The listing builds one solid part. Answer for the finished solid, in the listing's coordinates (mm). Face numbers are marked on the shaded views. A direction names the side the tool comes from. Round coordinates to 2 decimals unless told otherwise and drop trailing zeros. Write each loop counter-clockwise with the first axis right and the second up, starting at its lowest first coordinate (ties: lowest second). Pieces come first, ordered by that corner, then holes.
Item 1: For a pull along Z with two mould halves and no side action, classify the marked faces 3, 4 and 5 as +Z half, -Z half, draft (parallel to the pull), parting line (faces both ways), or undercut.
Item 2: Find section D-D on z = -3.5. Give the vertices of the cut face in (x, y), then the cut area to 3 significant figures.
Item 3: Find section C-C on x = 13. Give the vertices of the cut face in (y, z), then the cut area to 3 significant figures.
Item 4: Find section A-A on z = 0. Give the vertices of the cut face in (x, y) (3 decimals).
Item 5: Each of these flat-tipped pins is pushed along its axis until it touches: pin 1 (3 mm diameter, centred on y = 2.5, z = 3.5, fed in from -X); pin 2 (2 mm diameter, centred on x = 6.5, z = -2, fed in from +Y). Where does it stop, or does it pass through?
Item 6: A tool of negligible diameter and unlimited length cuts with its end or side. For the marked faces 1 and 2, from which of +Z, -Z, +X, -X, +Y, -Y can it reach the whole face along a straight path? Write none if from no direction.
Item 7: Find the intervals of material crossed by probe 1 along X at (y, z) = (3.3, 0) (3 decimals); probe 2 along Y at (x, z) = (9, -3); probe 3 along X at (y, z) = (4.25, -1.75), in increasing order.
Item 8: Find section B-B on y = 3.55. Give the vertices of the cut face in (x, z) (3 decimals).
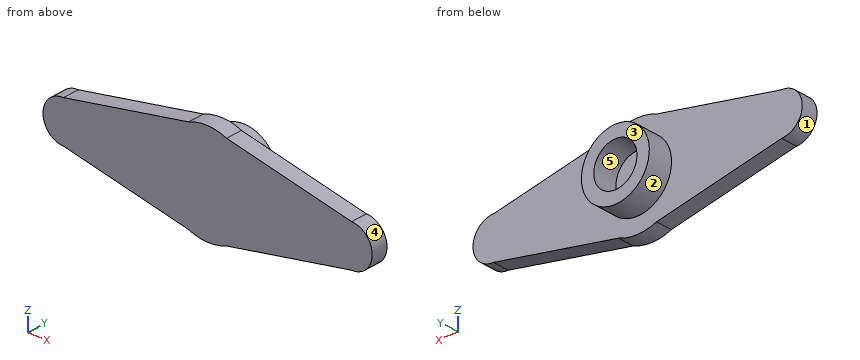
```python
from build123d import *

# Parameters (mm, degrees)
BOSS_EXTRUDE1_DEPTH = 2
SKETCH2_R           = 4.125
SKETCH2_R_2         = 2.625
BOSS_EXTRUDE2_DEPTH = 3


with BuildPart() as part:
    # Sketch1 → Boss-Extrude1 (new body)
    with BuildSketch(Plane(origin=(0, 0, 0), x_dir=(1, 0, 0), z_dir=(0, 1, 0))):
        with BuildLine():
            Line((17.5, 2.5), (2.307692308, 5.538461538))
            ThreePointArc((2.307692308, 5.538461538), (0, 6), (-2.307692308, 5.538461538))
            Line((-2.307692308, 5.538461538), (-17.5, 2.5))
            ThreePointArc((-17.5, 2.5), (-20, 0), (-17.5, -2.5))
            Line((-17.5, -2.5), (-2.307692308, -5.538461538))
            ThreePointArc((-2.307692308, -5.538461538), (0, -6), (2.307692308, -5.538461538))
            Line((2.307692308, -5.538461538), (17.5, -2.5))
            ThreePointArc((17.5, -2.5), (20, 0), (17.5, 2.5))
        make_face()
    extrude(amount=BOSS_EXTRUDE1_DEPTH)

    # Sketch2 → Boss-Extrude2 (add)
    with BuildSketch(Plane(origin=(0, 2, 0), x_dir=(1, 0, 0), z_dir=(0, 1, 0))):
        with Locations(Location((0, 0, 0), (0, 0, 270))):
            Circle(SKETCH2_R)
        with Locations(Location((0, 0, 0), (0, 0, 270))):
            Circle(SKETCH2_R_2, mode=Mode.SUBTRACT)
    extrude(amount=BOSS_EXTRUDE2_DEPTH)


solid = part.part
```
Check values:
1. face 3: draft
1. face 4: parting line
1. face 5: undercut
2. outline: (-12.5, 0) - (12.5, 0) - (12.5, 2) - (2.18, 2) - (2.18, 5) - (-2.18, 5) - (-2.18, 2) - (-12.5, 2) - close
2. area: 63.1 mm2
3. outline: (0, -3.4) - (2, -3.4) - (2, 3.4) - (0, 3.4) - close
3. area: 13.6 mm2
4. outline: (-20, 0) - (20, 0) - (20, 2) - (4.125, 2) - (4.125, 5) - (2.625, 5) - (2.625, 2) - (-2.625, 2) - (-2.625, 5) - (-4.125, 5) - (-4.125, 2) - (-20, 2) - close
5. pin 1: stops at x = -18.88
5. pin 2: stops at y = 2
6. face 1: -X, +Y, -Y
6. face 2: +Y
7. probe 1: x = -4.125 to -2.625, 2.625 to 4.125
7. probe 2: y = 0 to 2
7. probe 3: x = -3.74 to -1.96, 1.96 to 3.74
8. outline: circle Ø8.25 at (0, 0); hole circle Ø5.25 at (0, 0)
